from build123d import *

# Parameters (mm, degrees)
BOSS_EXTRUDE1_DEPTH = 2.9
SKETCH3_R           = 0.675
CUT_EXTRUDE1_DEPTH  = 3
LPATTERN1_COUNT     = 12
LPATTERN1_PITCH     = 2.54


with BuildPart() as part:
    # Sketch2 → Boss-Extrude1 (new body)
    with BuildSketch(Plane(origin=(0, 0, 0), x_dir=(1, 0, 0), z_dir=(0, 1, 0))):
        Polygon((-1.02, 1.27), (1.02, 1.27), (1.27, 1.02), (1.27, -1.02), (1.02, -1.27), (-1.02, -1.27), (-1.27, -1.02), (-1.27, 1.02), align=None)
    boss_extrude1 = extrude(amount=BOSS_EXTRUDE1_DEPTH)

    # Sketch3 → Cut-Extrude1 (cut)
    with BuildSketch(Plane(origin=(0, 2.9, 0), x_dir=(1, 0, 0), z_dir=(0, 1, 0))):
        with Locations(Location((0, 0, 0), (0, 0, 270))):
            Circle(SKETCH3_R)
    cut_extrude1 = extrude(amount=-CUT_EXTRUDE1_DEPTH, mode=Mode.SUBTRACT)

    # LPattern1: Boss-Extrude1, Cut-Extrude1 ×12
    with Locations(*[(i * LPATTERN1_PITCH, 0, 0) for i in range(1, LPATTERN1_COUNT)]):
        add(boss_extrude1)
        add(cut_extrude1, mode=Mode.SUBTRACT)


solid = part.part
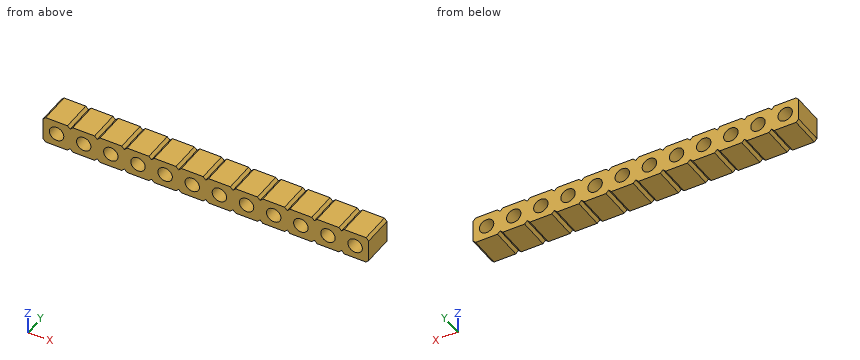
Read the model definition and answer for the solid it produces. Units are mm, in the model's axes. Round coordinates to 2 decimals unless told otherwise and drop trailing zeros. Order: outer loops, then holes, each group sorted by start corner. A loop starts at its lowest first (then second) coordinate and runs counter-clockwise, first axis right, second up. Notation, with made-up numbers: (4, -15) - (41, -15) arc R31 cw to (41, 23) - close; hole circle Ø8 at (11.5, 33). An arc over 180 degrees is marked (long way). Use one line per item in the form item = value. Start each with the question number.
(1) Find the intervals of material crossed by line 1 along Z through (x, y) = (0.5, 2.2); line 2 along Z through (x, y) = (5, 2.1); line 3 along Z through (x, y) = (1.5, 2.35), in increasing order. Write a range as from..to.
(2) The part is cut by section B-B (z = 0.2). Count the separate pieces of the cut face and the enclosed holes in it, then the cut area to 3 significant figures.
(3) The part is cut by section D-D (x = 13). Give the vertices of the cut face in (y, z), then the cut area to 3 significant figures.
(4) The part is cut by section A-A (x = 25.4). Give the vertices of the cut face in (y, z) (3 decimals), then the cut area to 3 significant figures.
(5) A flat-ended cylindrical pin translates along its axis: pin 1 Ø1.2 at (x, z) = (12.7, 0) entering from +Y. Find the tip coordinate at first contact, or state that the pin passes through.
Checked values:
q1.line_1 = -1.27..-0.45, 0.45..1.27
q1.line_2 = -1.27..-0.67, 0.67..1.27
q1.line_3 = -1.25..1.25
q2.separate_pieces = 13
q2.enclosed_holes = 0
q2.area = 43.5 mm^2
q3.outline = (0, -1.27) - (2.9, -1.27) - (2.9, -0.6) - (0, -0.6) - close; (0, 0.6) - (2.9, 0.6) - (2.9, 1.27) - (0, 1.27) - close
q3.area = 3.86 mm^2
q4.outline = (0, -1.27) - (2.9, -1.27) - (2.9, -0.675) - (0, -0.675) - close; (0, 0.675) - (2.9, 0.675) - (2.9, 1.27) - (0, 1.27) - close
q4.area = 3.45 mm^2
q5.pin_1 = through
